Build history of the part. All positions in model axes, mm. A direction names the side the tool comes from. Round coordinates to 2 decimals unless told otherwise and drop trailing zeros. Loops run counter-clockwise (first coordinate to the right, second up) from the corner with the lowest first, then second, coordinate; pieces in that order, holes last. Notation, with made-up numbers: (-23.75, 57.5) - (-17.75, 57.5) arc R12 cw to (-17.75, 61.5) - close; hole circle Ø8 at (83.25, 7). An arc over 180 degrees is marked (long way). Answer as CSV lines item,"result". Start each with the question number.
```python
from build123d import *

# Parameters (mm, degrees)
SKETCH1_W               = 13.97
SKETCH1_H               = 2.38125
CUT_EXTRUDE1_DEPTH      = 32.597232474
CUT_EXTRUDE1_DEPTH_BACK = 32.597232474
SKETCH2_R               = 1.5
CUT_EXTRUDE2_DEPTH      = 1.27
CHAMFER1_SIZE           = 6.35


with BuildPart() as part:
    # Sketch1 → Revolve1 (revolve)
    with BuildSketch(Plane.XY, mode=Mode.PRIVATE) as revolve1_sk:
        with Locations((6.985, 4.454525)):
            Rectangle(SKETCH1_W, SKETCH1_H)
        Polygon((13.97, 5.64515), (13.97, 3.2639), (16.51, 3.2639), (16.51, 19.05), (13.97, 19.05), align=None)
        with Locations((-6.985, 4.454525)):
            Rectangle(SKETCH1_W, SKETCH1_H)
        Polygon((-16.51, 3.2639), (-13.97, 3.2639), (-13.97, 5.64515), (-13.97, 19.05), (-16.51, 19.05), align=None)
    revolve(revolve1_sk.sketch.rotate(Axis((-15.275524476, 0, 0), (1, 0, 0)), 90), axis=Axis((-15.275524476, 0, 0), (1, 0, 0)))

    # Sketch2 → Cut-Extrude1 (cut, two sides: drawn at the far end of the back side and taken through both)
    with BuildSketch(Plane(origin=(0, 0, 0), x_dir=(1, 0, 0), z_dir=(0, 1, 0)).offset(-CUT_EXTRUDE1_DEPTH_BACK)):
        with Locations(Location((0, 0, 0), (0, 0, 90))):
            Circle(SKETCH2_R)
    extrude(amount=CUT_EXTRUDE1_DEPTH + CUT_EXTRUDE1_DEPTH_BACK, mode=Mode.SUBTRACT)

    # Sketch3 → Cut-Extrude2 (cut)
    with BuildSketch(Plane(origin=(16.51, 0, 0), x_dir=(0, 0, -1), z_dir=(1, 0, 0))):
        with BuildLine():
            Line((-0.892975977, 11.138058786), (-1.272890507, 11.138058786))
            add(Edge.make_bspline(
                [(-1.272890507, 11.138058786), (-1.262598003, 11.180673314), (-1.242476999, 11.263981231), (-1.200509458, 11.383007156), (-1.154790359, 11.495642272), (-1.099891156, 11.599777524), (-1.040009139, 11.69750572), (-0.971401657, 11.78661028), (-0.897233992, 11.869357391), (-0.815198101, 11.942791497), (-0.729166292, 12.00928837), (-0.637926323, 12.065984868), (-0.543313871, 12.114757891), (-0.444673415, 12.154938552), (-0.341711283, 12.185207519), (-0.23535831, 12.207168607), (-0.125335791, 12.221430241), (-0.05065061, 12.222822116), (-0.01272758, 12.223528871)],
                knots=[0, 0, 0, 0, 1.162005537, 2.271625781, 3.343758855, 4.383309926, 5.390229558, 6.379919256, 7.361854164, 8.333198761, 9.295911338, 10.242430842, 11.177959212, 12.116337295, 13.062827104, 14.020064771, 14.994644689, 16, 16, 16, 16], degree=3))
            add(Edge.make_bspline(
                [(-0.01272758, 12.223528871), (0.042526785, 12.221860659), (0.151830255, 12.218560624), (0.312410321, 12.18842602), (0.467261807, 12.140740384), (0.614689755, 12.074853114), (0.751630144, 11.993588459), (0.873472961, 11.896869206), (0.978566683, 11.786561479), (1.066734169, 11.664723044), (1.135767739, 11.534511142), (1.18667221, 11.400495714), (1.217662243, 11.262994663), (1.221678536, 11.170154906), (1.22369069, 11.123642386)],
                knots=[0, 0, 0, 0, 1.083050992, 2.142477498, 3.193116406, 4.255571735, 5.30263384, 6.308962982, 7.297363603, 8.282367274, 9.249857812, 10.179914175, 11.08814088, 12, 12, 12, 12], degree=3))
            add(Edge.make_bspline(
                [(1.22369069, 11.123642386), (1.222283298, 11.078881787), (1.219529252, 10.99129224), (1.196144675, 10.863419572), (1.156791291, 10.742900684), (1.10227834, 10.629228231), (1.031712846, 10.523122948), (0.946232536, 10.424346109), (0.845234078, 10.332459603), (0.768696696, 10.279821765), (0.729292987, 10.252722247)],
                knots=[0, 0, 0, 0, 1.024540389, 2.004866551, 2.965041327, 3.920577974, 4.882998113, 5.874504559, 6.905732034, 8, 8, 8, 8], degree=3))
            add(Edge.make_bspline(
                [(0.729292987, 10.252722247), (0.77432568, 10.230977221), (0.863548471, 10.187894034), (0.98516673, 10.103401832), (1.095569494, 10.005846059), (1.157138754, 9.929715422), (1.188073702, 9.891464234)],
                knots=[0, 0, 0, 0, 1.015518401, 2.012035669, 3.001164323, 4, 4, 4, 4], degree=3))
            add(Edge.make_bspline(
                [(1.188073702, 9.891464234), (1.208443707, 9.863575335), (1.248850143, 9.808254236), (1.298725503, 9.719310178), (1.343972717, 9.629380281), (1.379230602, 9.536054143), (1.406534231, 9.44041345), (1.426051146, 9.34229398), (1.438175583, 9.24161561), (1.439911918, 9.173504325), (1.440784707, 9.139267386)],
                knots=[0, 0, 0, 0, 1.025084078, 2.033381695, 3.024893161, 4.013698104, 4.991890475, 5.976764909, 6.982997093, 8, 8, 8, 8], degree=3))
            add(Edge.make_bspline(
                [(1.440784707, 9.139267386), (1.4386142, 9.079988962), (1.434283401, 8.961711077), (1.395573711, 8.786965462), (1.335565315, 8.616149854), (1.250345973, 8.45277362), (1.146487177, 8.29991354), (1.022925461, 8.163145052), (0.881064757, 8.045581026), (0.722852211, 7.947355321), (0.55144197, 7.868835549), (0.368107682, 7.814337499), (0.17549095, 7.778842814), (0.043402124, 7.775036601), (-0.023751885, 7.773101521)],
                knots=[0, 0, 0, 0, 0.955779014, 1.907060117, 2.875433937, 3.871313158, 4.872415639, 5.851225146, 6.836215519, 7.83643374, 8.849228613, 9.86973379, 10.916971861, 12, 12, 12, 12], degree=3))
            add(Edge.make_bspline(
                [(-0.023751885, 7.773101521), (-0.06901142, 7.774151645), (-0.158067092, 7.77621794), (-0.28899018, 7.790343487), (-0.413960236, 7.816142636), (-0.533146225, 7.850859967), (-0.646654031, 7.894876646), (-0.754137282, 7.94969069), (-0.856257249, 8.014172221), (-0.952050266, 8.08908237), (-1.041504915, 8.1728798), (-1.122243924, 8.267052126), (-1.195613388, 8.36985851), (-1.25964877, 8.482493064), (-1.317266798, 8.603500185), (-1.364657098, 8.734429321), (-1.406368214, 8.874109995), (-1.425761071, 8.971449738), (-1.43571102, 9.021392119)],
                knots=[0, 0, 0, 0, 1.048658725, 2.063410685, 3.046034179, 4.001477787, 4.936774919, 5.862367409, 6.792675028, 7.730719943, 8.675894397, 9.627829632, 10.600096036, 11.597688215, 12.626045268, 13.701542398, 14.82072376, 16, 16, 16, 16], degree=3))
            Line((-1.43571102, 9.021392119), (-1.05579649, 9.021392119))
            add(Edge.make_bspline(
                [(-1.05579649, 9.021392119), (-1.045898604, 8.988796646), (-1.026646356, 8.925395619), (-0.993875158, 8.834148773), (-0.956539248, 8.750500461), (-0.916486401, 8.673837066), (-0.874421042, 8.603403589), (-0.827352514, 8.541062471), (-0.778766976, 8.484075512), (-0.742143377, 8.451969172), (-0.7242193, 8.436255901)],
                knots=[0, 0, 0, 0, 1.198163088, 2.33053128, 3.407730985, 4.417276592, 5.372219308, 6.28897303, 7.162600585, 8, 8, 8, 8], degree=3))
            add(Edge.make_bspline(
                [(-0.7242193, 8.436255901), (-0.700516774, 8.417982012), (-0.653184886, 8.38149064), (-0.576055693, 8.334922003), (-0.494939116, 8.294571049), (-0.408077558, 8.263747912), (-0.317345407, 8.237649218), (-0.221276117, 8.220570114), (-0.120717255, 8.20885204), (-0.052055293, 8.20781798), (-0.016967697, 8.207289555)],
                knots=[0, 0, 0, 0, 0.946170439, 1.889420265, 2.845303464, 3.807233317, 4.801018734, 5.828864929, 6.890507805, 8, 8, 8, 8], degree=3))
            add(Edge.make_bspline(
                [(-0.016967697, 8.207289555), (0.022648444, 8.208034507), (0.100114388, 8.209491196), (0.213150266, 8.222887528), (0.320685941, 8.242397647), (0.421527479, 8.272530493), (0.516995807, 8.309760665), (0.60575266, 8.356506832), (0.688963188, 8.411352352), (0.765561612, 8.473690192), (0.834438559, 8.541933334), (0.895083494, 8.613311048), (0.946639037, 8.687522385), (0.988226794, 8.764978017), (1.021066031, 8.845357198), (1.043421902, 8.928885497), (1.058966115, 9.014879333), (1.060232018, 9.073334372), (1.060870177, 9.102802376)],
                knots=[0, 0, 0, 0, 1.217147791, 2.380027433, 3.494444702, 4.572153297, 5.609568379, 6.639424714, 7.649109417, 8.668170816, 9.669597737, 10.625200337, 11.543417969, 12.441394052, 13.322311151, 14.205496177, 15.095365482, 16, 16, 16, 16], degree=3))
            add(Edge.make_bspline(
                [(1.060870177, 9.102802376), (1.059019241, 9.142246566), (1.055326578, 9.220938679), (1.027134296, 9.336711364), (0.980762527, 9.448257777), (0.915844347, 9.553674781), (0.836819228, 9.651375157), (0.744454055, 9.738547331), (0.637981816, 9.810477822), (0.539986356, 9.86017553), (0.45318469, 9.89408704), (0.378901321, 9.916674854), (0.295738572, 9.935801847), (0.204702131, 9.95359669), (0.10510605, 9.968741559), (-0.002941242, 9.981371183), (-0.119461639, 9.991476804), (-0.200126192, 9.995989653), (-0.241693926, 9.998315196)],
                knots=[0, 0, 0, 0, 1.07054697, 2.135767047, 3.216561865, 4.33974944, 5.486079747, 6.621378074, 7.775625952, 8.963672916, 9.598146892, 10.304877434, 11.070270905, 11.915000392, 12.823868403, 13.805723172, 14.86925407, 16, 16, 16, 16], degree=3))
            Line((-0.241693926, 9.998315196), (-0.241693926, 10.43250323))
            add(Edge.make_bspline(
                [(-0.241693926, 10.43250323), (-0.189320135, 10.433391993), (-0.086732744, 10.43513286), (0.063120367, 10.456188263), (0.206416659, 10.485314356), (0.339980433, 10.529927875), (0.461717448, 10.581744234), (0.567332586, 10.642041668), (0.655346183, 10.709067127), (0.725330526, 10.78385514), (0.777980165, 10.864064769), (0.816475434, 10.947663012), (0.839214876, 11.03538259), (0.842250378, 11.09524757), (0.84377616, 11.125338433)],
                knots=[0, 0, 0, 0, 1.321986639, 2.589447074, 3.816329219, 5.01088745, 6.139805852, 7.153945165, 8.075214402, 8.924034688, 9.728124013, 10.488707548, 11.240355623, 12, 12, 12, 12], degree=3))
            add(Edge.make_bspline(
                [(0.84377616, 11.125338433), (0.84327492, 11.147445801), (0.842277727, 11.191427361), (0.829701972, 11.255683397), (0.810804322, 11.317975017), (0.784824078, 11.378037321), (0.750050028, 11.435453747), (0.708435168, 11.490713805), (0.658883276, 11.543501994), (0.60210164, 11.592705809), (0.541127361, 11.639598125), (0.474301443, 11.679407952), (0.403638794, 11.713450075), (0.329061183, 11.741522521), (0.250326589, 11.762639945), (0.167804944, 11.777802344), (0.081338888, 11.787282174), (0.022348317, 11.78864702), (-0.007639439, 11.789340837)],
                knots=[0, 0, 0, 0, 0.884392785, 1.759457502, 2.611959086, 3.489218968, 4.37281399, 5.2945488, 6.255912374, 7.266815255, 8.301784654, 9.332968512, 10.37626691, 11.440494194, 12.520033166, 13.637162961, 14.798855837, 16, 16, 16, 16], degree=3))
            add(Edge.make_bspline(
                [(-0.007639439, 11.789340837), (-0.05584098, 11.787657952), (-0.149989801, 11.784370885), (-0.285716415, 11.755580573), (-0.411893133, 11.709645177), (-0.508338949, 11.654813811), (-0.579558824, 11.600687096), (-0.630451883, 11.553416019), (-0.680430024, 11.500882984), (-0.726205271, 11.439852378), (-0.772498557, 11.374457308), (-0.814643884, 11.301373427), (-0.855597988, 11.222507159), (-0.880275358, 11.166753392), (-0.892975977, 11.138058786)],
                knots=[0, 0, 0, 0, 1.472543308, 2.876219568, 4.221790263, 5.565193594, 6.249813518, 6.953379497, 7.687249741, 8.463570142, 9.283606569, 10.136032583, 11.040678096, 12, 12, 12, 12], degree=3))
        make_face()
    extrude(amount=-CUT_EXTRUDE2_DEPTH, mode=Mode.SUBTRACT)

    # Chamfer1
    chamfer1_edges = [part.edges().sort_by_distance(p)[0] for p in [
        (-13.97, 0, -5.64515),
        (13.97, 0, -5.64515),
    ]]
    chamfer(chamfer1_edges, length=CHAMFER1_SIZE)


solid = part.part
```
Q1. Band-saw the part on C-C, the plane x = 4.5. List the corners of the cut face in (y, z), then the cut area to 3 significant figures.
Q2. Pin check, flat tips, straight feed: pin 1 Ø10 at (x, y) = (6, 2) entering from +Z; pin 2 Ø6 at (x, z) = (-4, -3) entering from +Y; pin 3 Ø2 at (x, z) = (-0.5, -3) entering from +Y. Stop position of each tip, or through.
Q3. Wall check: probe 1 along X at (y, z) = (-2, 14.5); probe 2 along Y at (x, z) = (4, 0); probe 3 along Y at (x, z) = (9, 0). Give the ranges that are in metal, low to high. Write a range as [from, to].
Q4. Band-saw the part on B-B, the plane y = 14.5. List the corners of the cut face in (x, z).
Q5. Band-saw the part on A-A, the plane x = 0. List the corners of the cut face in (y, z), then the cut area to 3 significant figures.
Q6. Two-plate mould, pull along Z, no slides. Class faces 1 (the conical face through (-8.017, -1.815, 5.763)), 2 (the flat face through (15.24, 10.2, -0.1)), 3 (the flat face through (13.97, 12.4, -0.3)): released by +Z, released by -Z, zero draft, split by the parting line, or undercut.
Q7. Tool access for faces 4 (the flat face through (-13.97, 12.4, 0.3)), 5 (the cylindrical face through (0.9, -4.3, 1.2)): list every direction of +Z, -Z, +X, -X, +Y, -Y with a clear straight run to the whole face (end or side of a thin tool).
Reported:
1,outline,"circle Ø11.29 at (0, 0); hole circle Ø6.53 at (0, 0)"
1,area,"66.6 mm2"
2,pin 1,"stops at z = 8.88"
2,pin 2,"stops at y = 5.65"
2,pin 3,"stops at y = 5.28"
3,probe 1,"x = [-16.51, -13.97], [13.97, 16.51]"
3,probe 2,"y = [-5.65, -3.26], [3.26, 5.65]"
3,probe 3,"y = [-7.03, -3.26], [3.26, 7.03]"
4,outline,"(-16.51, -12.36) - (-13.97, -12.36) - (-13.97, 12.36) - (-16.51, 12.36) - close; (13.97, -12.36) - (16.51, -12.36) - (16.51, 12.36) - (13.97, 12.36) - close"
5,outline,"(-5.44, -1.5) arc R5.65 ccw to (5.44, -1.5) - (2.9, -1.5) arc R3.26 cw to (-2.9, -1.5) - close; (-5.44, 1.5) - (-2.9, 1.5) arc R3.26 cw to (2.9, 1.5) - (5.44, 1.5) arc R5.65 ccw to start"
5,area,"52.1 mm2"
6,face 1,"split by the parting line"
6,face 2,"undercut"
6,face 3,"zero draft"
7,face 4,"none"
7,face 5,"+Y, -Y"
